Could you check a few things on this model? Use its own coordinates, in mm. Face numbers are marked on the shaded views. A direction names the side the tool comes from. Give positions to 0.01 mm unless a question says otherwise; leave off trailing zeros. Write each loop counter-clockwise with the first axis right and the second up, starting at its lowest first coordinate (ties: lowest second). Pieces come first, ordered by that corner, then holes. Notation, with made-up numbers: (-30, 5.25) -> (-1, 5.25) arc R21 cw to (-1, 32.25) -> close; hole circle Ø11 at (24.25, 65). An arc over 180 degrees is marked (long way). Write item = value, one per line. Start each with the question number.
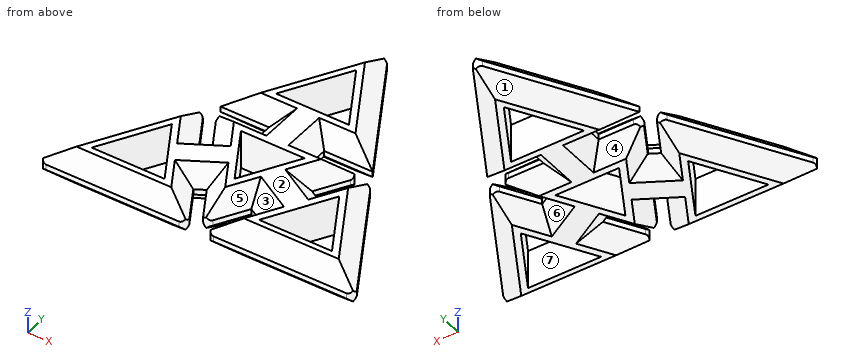
```python
from build123d import *

# Parameters (mm, degrees)
F0_W     = 5
F0_H     = 2
F1_DEPTH = 3.5
F2_SIZE  = 3
F3_R     = 1
F6_DEPTH = 9.2


with BuildPart() as f1:
    # F0 (on Top) → F1 (new body)
    with BuildSketch(Plane.XY):
        Polygon((-4.0418434781, -8.107062112), (0, -15.1077403724), (0, 7.5538701862), (-5, 7.5538701862), (-13.0836869563, 7.5538701862), (-9.0418434781, 0.5531919258), (-6.5418434781, -3.7769350931), align=None)
        Polygon((0, 7.5538701862), (0, -15.1077403724), (4.0418434781, -8.107062112), (6.5418434781, -3.7769350931), (9.0418434781, 0.5531919258), (13.0836869563, 7.5538701862), (5, 7.5538701862), align=None)
        Polygon((-10.7738942857, -0.4468080742), (-8.2738942857, -4.7769350931), (-6.5418434781, -3.7769350931), (-9.0418434781, 0.5531919258), align=None)
        Polygon((-8.2738942857, -4.7769350931), (-5.7738942857, -9.107062112), (-4.0418434781, -8.107062112), (-6.5418434781, -3.7769350931), align=None)
        Polygon((8.2738942857, -4.7769350931), (10.7738942857, -0.4468080742), (9.0418434781, 0.5531919258), (6.5418434781, -3.7769350931), align=None)
        Polygon((4.0418434781, -8.107062112), (5.7738942857, -9.107062112), (8.2738942857, -4.7769350931), (6.5418434781, -3.7769350931), align=None)
        with Locations((2.5, 8.5538701862)):
            Rectangle(F0_W, F0_H)
        with Locations((-2.5, 8.5538701862)):
            Rectangle(F0_W, F0_H)
        Polygon((-28.9386550611, -16.7077402895), (-1.3856406939, -16.7077402895), (-5.7738942857, -9.107062112), (-8.2738942857, -4.7769350931), (-10.7738942857, -0.4468080742), (-15.1621478775, 7.1538701033), align=None)
        Polygon((5.7738942857, -9.107062112), (1.3856406939, -16.7077402895), (28.9386550611, -16.7077402895), (15.1621478775, 7.1538701033), (10.7738942857, -0.4468080742), (8.2738942857, -4.7769350931), align=None)
        Polygon((5, 9.5538701862), (13.7765071836, 9.5538701862), (0, 33.415480579), (0, 9.5538701862), align=None)
        Polygon((0, 9.5538701862), (0, 33.415480579), (-13.7765071836, 9.5538701862), (-5, 9.5538701862), align=None)
    extrude(amount=F1_DEPTH)

    # F2
    f2_edges = [f1.edges().sort_by_distance(p)[0] for p in [
        (-11.062765, 4.053531, 3.5),
        (-9.907869, 0.053192, 3.5),
        (-12.968021, 3.353531, 3.5),
        (-22.050401, -4.776935, 3.5),
        (-15.162148, -16.70774, 3.5),
        (-3.579767, -12.907401, 3.5),
        (-4.907869, -8.607062, 3.5),
        (-2.020922, -11.607401, 3.5),
        (2.020922, -11.607401, 3.5),
        (4.907869, -8.607062, 3.5),
        (3.579767, -12.907401, 3.5),
        (15.162148, -16.70774, 3.5),
        (22.050401, -4.776935, 3.5),
        (12.968021, 3.353531, 3.5),
        (9.907869, 0.053192, 3.5),
        (11.062765, 4.053531, 3.5),
        (9.041843, 7.55387, 3.5),
        (5, 8.55387, 3.5),
        (9.388254, 9.55387, 3.5),
        (6.888254, 21.484675, 3.5),
        (-6.888254, 21.484675, 3.5),
        (-9.388254, 9.55387, 3.5),
        (-5, 8.55387, 3.5),
        (-9.041843, 7.55387, 3.5),
    ]]
    chamfer(f2_edges, length=F2_SIZE)

    # F3
    f3_edges = [f1.edges().sort_by_distance(p)[0] for p in [
        (-28.938655, -16.70774, 0.25),
        (28.938655, -16.70774, 0.25),
        (0, 33.415481, 0.25),
        (-15.162148, 7.15387, 0.25),
        (15.162148, 7.15387, 0.25),
        (-1.385641, -16.70774, 0.25),
        (1.385641, -16.70774, 0.25),
        (-13.083687, 7.55387, 0.25),
        (13.083687, 7.55387, 0.25),
        (0, -15.10774, 0.25),
    ]]
    fillet(f3_edges, radius=F3_R)

    # F4: F1 across plane


with BuildPart() as f1_1:
    add(f1.part)
    add(f1.part.mirror(Plane.XY))

    # F5 (on face) → F6 (cut)
    with BuildSketch(Plane.XY.offset(3.5)):
        Polygon((-6.6051743925, 13.6882647859), (6.6051743925, 13.6882647859), (0, 25.1287624265), align=None)
        Polygon((-21.7569312081, -12.6255113644), (-8.5465824232, -12.6255113644), (-15.1517568156, -1.1850137238), align=None)
        Polygon((8.6276847869, -12.7216648323), (21.8380335718, -12.7216648323), (15.2328591794, -1.2811671917), align=None)
        Polygon((-5.7627101947, 3.3271022821), (0, -6.6542045643), (5.7627101947, 3.3271022821), align=None)
    extrude(amount=-F6_DEPTH, mode=Mode.SUBTRACT)


solid = f1_1.part
```
(1) Imagine slicing it at A-A (x = -17). Please give me the cut outline in (y, z), then the cut area to 3 significant figures.
(2) I'm going to push flat-ended pins straight in: pin 1 (0.5 mm diameter, centred on x = -8.5, z = 0, fed in from +Y); pin 2 (0.8 mm diameter, centred on x = 8, z = 0, fed in from +Y); pin 3 (0.8 mm diameter, centred on y = 9, z = 0, fed in from +X). Where does each tip first touch, or does it pass through?
(3) On a 3-axis mill with a long thin cutter (end or side, diameter ignored), from which of +Z, -Z, +X, -X, +Y, -Y can I reach the whole of each face in a straight line? I mean the marked faces 4, 5, 6 and 7. Say none if no direction works.
(4) If I drill on line 1 along Y through (x, z) = (-5.5, -1); line 2 along X through (y, z) = (3, 1); line 3 along Y through (x, z) = (2, -0.25), over which ranges is the centre line in solid material (lowest first)? Write a range as from..to.
(5) We'd pull the mould along Y, two halves only. Please class the marked faces 1, 2 and 3: released by +Y, released by -Y, zero draft, split by the parting line, or undercut.
(6) Imagine slicing it at B-B (y = -6). State how many separate pieces and enclosed holes the cut face has, then the cut area to 3 significant figures.
Answers below:
q1.outline = (-16.71, -0.5) -> (-13.71, -3.5) -> (-12.63, -3.5) -> (-12.63, 3.5) -> (-13.71, 3.5) -> (-16.71, 0.5) -> close; (-4.39, -3.5) -> (-2.03, -3.5) -> (3.97, -0.5) -> (3.97, 0.5) -> (-2.03, 3.5) -> (-4.39, 3.5) -> close
q1.area = 60.1 mm^2
q2.pin_1 = 19.13
q2.pin_2 = 20.25
q2.pin_3 = 5
q3.face_4 = -Z, -X
q3.face_5 = +Z
q3.face_6 = -Z
q3.face_7 = +Z, -Z
q4.line_1 = -16.21..-10.58, -8.37..2.87, 3.33..7.05, 10.05..13.69, 15.6..22.89
q4.line_2 = -16.98..-13.34, -9.88..-5.57, 5.57..9.88, 13.34..16.98
q4.line_3 = -11.64..-3.19, 3.33..13.69, 21.66..29.95
q5.face_1 = released by +Y
q5.face_2 = zero draft
q5.face_3 = undercut
q6.separate_pieces = 4
q6.enclosed_holes = 0
q6.area = 202 mm^2
